Here's how the part is built. I have some questions about the finished solid (model axes, mm). Face numbers are marked on the shaded views. A direction names the side the tool comes from. Coordinates: 2 decimals unless noted, no trailing zeros. Order: outer loops, then holes, each group sorted by start corner. A loop starts at its lowest first (then second) coordinate and runs counter-clockwise, first axis right, second up. Notation, with made-up numbers: (9, 23.5) -> (45, 23.5) arc R16 cw to (45, 33.5) -> close; hole circle Ø7 at (23.5, 70). An arc over 180 degrees is marked (long way). One line per item, written item: value. Start each with the question number.
```python
from build123d import *

# Parameters (mm, degrees)
SKETCH1_R           = 19
BOSS_EXTRUDE1_DEPTH = 130
SKETCH2_R           = 19
SKETCH2_R_2         = 12.5
CUT_EXTRUDE2_DEPTH  = 35
SKETCH3_R           = 19
SKETCH3_R_2         = 12.5
CUT_EXTRUDE3_DEPTH  = 35
FILLET1_R           = 2.5


with BuildPart() as part:
    # Sketch1 → Boss-Extrude1 (new body)
    with BuildSketch(Plane.XY):
        Circle(SKETCH1_R)
    extrude(amount=BOSS_EXTRUDE1_DEPTH)

    # Sketch2 → Cut-Extrude2 (cut)
    with BuildSketch(Plane.XY.offset(130)):
        Circle(SKETCH2_R)
        Circle(SKETCH2_R_2, mode=Mode.SUBTRACT)
    extrude(amount=-CUT_EXTRUDE2_DEPTH, mode=Mode.SUBTRACT)

    # Sketch3 → Cut-Extrude3 (cut)
    with BuildSketch(Plane(origin=(0, 0, 0), x_dir=(-1, 0, 0), z_dir=(0, 0, -1))):
        Circle(SKETCH3_R)
        Circle(SKETCH3_R_2, mode=Mode.SUBTRACT)
    extrude(amount=-CUT_EXTRUDE3_DEPTH, mode=Mode.SUBTRACT)

    # Fillet1
    fillet1_edges = [part.edges().sort_by_distance(p)[0] for p in [
        (12.5, 0, 35),
        (-12.5, 0, 95),
    ]]
    fillet(fillet1_edges, radius=FILLET1_R)


solid = part.part
```
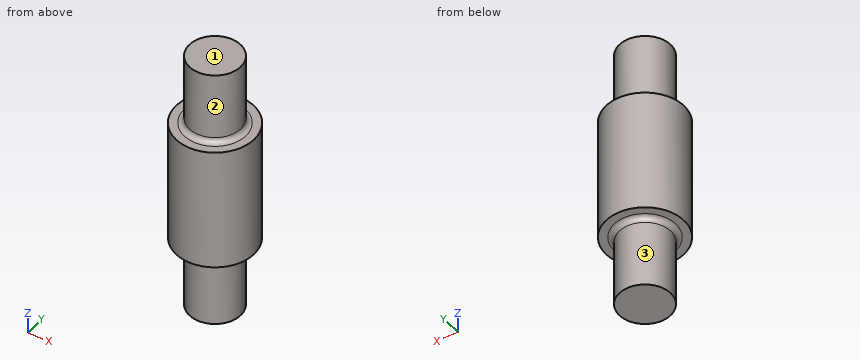
Q1. For P1, Ø2, axis at x = -3.5, z = 90, coming from the +Y side; P2, Ø1.5, axis at y = 4, z = 107.5, coming from the -X side; P3, Ø4, axis at y = 5, z = 73, coming from the +X side, each with a flat end and sliding along its axis, tell me the tip position at first contact or that it passes through.
Q2. For the marked faces 1, 2 and 3, which set-ups out of +Z, -Z, +X, -X, +Y, -Y let a thin tool reach every point of the face, with its end or its side?
Q3. I need wall thicknesses on line 1 (Z direction, x = -17, y = 6); line 2 (X direction, y = -8, z = 35.5); line 3 (Y direction, x = -7, z = 72.5). Which ranges of each line are inside material? Lowest first, please.
Q4. Imagine slicing it at D-D (z = 69.5). Write out the boundary of the cut face in (x, y), plus the area to 3 significant figures.
Q5. Imagine slicing it at C-C (z = 99.5). Write out the boundary of the cut face in (x, y).
Q6. Imagine slicing it at A-A (y = 0). Write out the boundary of the cut face in (x, z).
Completed:
1. P1: stops at y = 18.83
1. P2: stops at x = -12.07
1. P3: stops at x = 18.76
2. face 1: +Z, +X, -X, +Y, -Y
2. face 2: +Z
2. face 3: -Z
3. line 1: z = 35 to 95
3. line 2: x = -17.23 to 17.23
3. line 3: y = -17.66 to 17.66
4. outline: circle Ø38 at (0, 0)
4. area: 1,130 mm2
5. outline: circle Ø25 at (0, 0)
6. outline: (-19, 35) -> (-15, 35) arc R2.5 cw to (-12.5, 32.5) -> (-12.5, 0) -> (12.5, 0) -> (12.5, 32.5) arc R2.5 cw to (15, 35) -> (19, 35) -> (19, 95) -> (15, 95) arc R2.5 cw to (12.5, 97.5) -> (12.5, 130) -> (-12.5, 130) -> (-12.5, 97.5) arc R2.5 cw to (-15, 95) -> (-19, 95) -> close
